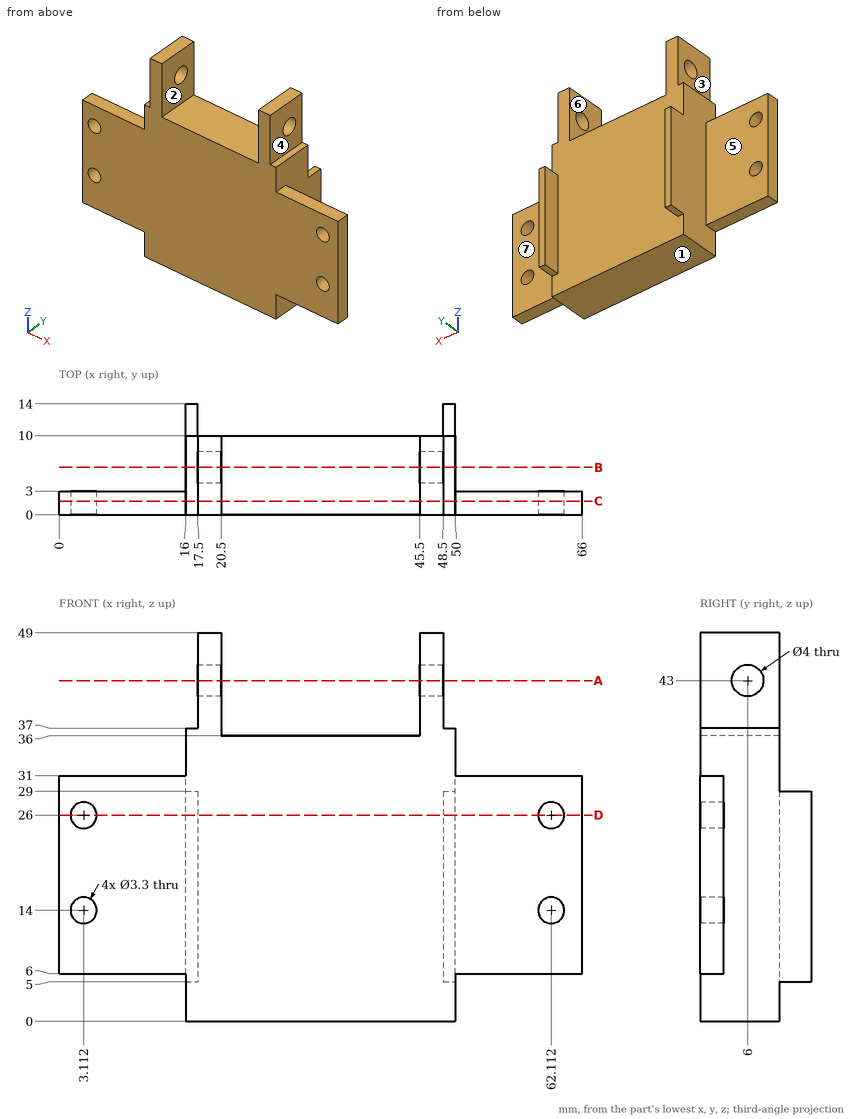
Verification items for this drawing (mm, ordinates from the low corner). A direction names the side the tool comes from. Give positions to 0.01 mm unless a question says otherwise; leave off trailing zeros. Write each loop counter-clockwise with the first axis right and the second up, starting at its lowest first coordinate (ties: lowest second). Pieces come first, ordered by that corner, then holes. Notation, with made-up numbers: (31, 2.5) - (76, 2.5) arc R14 ccw to (76, 11.5) - close; hole circle Ø4 at (66.25, 39). An arc over 180 degrees is marked (long way). Answer as a JSON object with one key per item and string values. Group by question number.
1) Sectioned sample at B-B (y = 6). Record the cut outline in (x, z), then the cut area to 3 significant figures.
2) Depth check by flat-ended pin: P1, Ø8, axis at x = 7.5, z = 24, coming from the +Y side; P2, Ø0.8, axis at x = 49, y = 5.5, coming from the +Z side; P3, Ø2.5, axis at x = 3.11, z = 14, coming from the +Y side; P4, Ø3.5, axis at x = 7, y = 1, coming from the +Z side. Enter the tip coordinate at first touch or a pass-through.
3) Sectioned sample at A-A (z = 43). Record the cut outline in (x, y).
4) Access from +Z, -Z, +X, -X, +Y, -Y to the whole of each face (thin tool, end or side, straight path). Record for the marked faces 5, 6 and 7.
5) Sectioned sample at D-D (z = 26). Record the cut outline in (x, y).
6) Thickness scan on probe 1 along X at (y, z) = (10.5, 25); probe 2 along Y at (x, z) = (18.3, 43); probe 3 along Y at (x, z) = (50.5, 15). Record the ranges inside material, lowest first. Write a range as from..to.
7) Sectioned sample at C-C (y = 1.75). Record the cut outline in (x, z).
8) Release check for a two-part mould opening along X. For the marked faces 1, 2, 3 and 4 record: pulls with the +X half, pulls with the -X half, needs draft (parallel to the pull), parting line crosses it, or undercut.
Geometry results:
{
 "1": {"outline": "(16, 0) - (50, 0) - (50, 37) - (48.5, 37) - (48.5, 41) - (45.5, 41) - (45.5, 36) - (20.5, 36) - (20.5, 41) - (17.5, 41) - (17.5, 37) - (16, 37) - close; (17.5, 45) - (20.5, 45) - (20.5, 49) - (17.5, 49) - close; (45.5, 45) - (48.5, 45) - (48.5, 49) - (45.5, 49) - close", "area": "1,280 mm^2"},
 "2": {"P1": "stops at y = 3", "P2": "stops at z = 37", "P3": "passes through", "P4": "stops at z = 31"},
 "3": {"outline": "(17.5, 0) - (20.5, 0) - (20.5, 4) - (17.5, 4) - close; (17.5, 8) - (20.5, 8) - (20.5, 10) - (17.5, 10) - close; (45.5, 0) - (48.5, 0) - (48.5, 4) - (45.5, 4) - close; (45.5, 8) - (48.5, 8) - (48.5, 10) - (45.5, 10) - close"},
 "4": {"face 5": "+Z, -Z, -X, +Y", "face 6": "+Z, +Y, -Y", "face 7": "+Z, -Z, +X, +Y"},
 "5": {"outline": "(0, 0) - (1.46, 0) - (1.46, 3) - (0, 3) - close; (4.76, 0) - (60.46, 0) - (60.46, 3) - (50, 3) - (50, 14) - (48.5, 14) - (48.5, 10) - (17.5, 10) - (17.5, 14) - (16, 14) - (16, 3) - (4.76, 3) - close; (63.76, 0) - (66, 0) - (66, 3) - (63.76, 3) - close"},
 "6": {"probe 1": "x = 16..17.5, 48.5..50", "probe 2": "y = 0..4, 8..10", "probe 3": "y = 0..3"},
 "7": {"outline": "(0, 6) - (16, 6) - (16, 0) - (50, 0) - (50, 6) - (66, 6) - (66, 31) - (50, 31) - (50, 37) - (48.5, 37) - (48.5, 49) - (45.5, 49) - (45.5, 36) - (20.5, 36) - (20.5, 49) - (17.5, 49) - (17.5, 37) - (16, 37) - (16, 31) - (0, 31) - close; hole circle Ø3.3 at (3.11, 14); hole circle Ø3.3 at (3.11, 26); hole circle Ø3.3 at (62.11, 14); hole circle Ø3.3 at (62.11, 26)"},
 "8": {"face 1": "needs draft", "face 2": "undercut", "face 3": "pulls with the -X half", "face 4": "pulls with the +X half"}
}
